The model under review builds one solid part; all positions refer to its coordinate system, in mm. A direction names the side the tool comes from. Give positions to 0.01 mm unless a question says otherwise; leave off trailing zeros. Order: outer loops, then holes, each group sorted by start corner. A loop starts at its lowest first (then second) coordinate and runs counter-clockwise, first axis right, second up. Notation, with made-up numbers: (25.5, 86) - (77.5, 86) arc R28 cw to (77.5, 107) - close; hole circle Ø7 at (69, 67.25). An arc over 180 degrees is marked (long way). Write item = value, one per line. Start each with the question number.
1. Machinability: for faces 5 (the flat face through (20, -31.2, 29)), 6 (the flat face through (14, -76, 0)), 7 (the flat face through (2, -37, 23.3)), 8 (the cylindrical face through (13.619, -62.627, 0.051)), 9 (the flat face through (17, 27, 28)), which of the approach directions +Z, -Z, +X, -X, +Y, -Y give a long, thin tool a straight path to every point of the face, cutting with its end or side? Answer none if there is none.
2. We need section B-B, the plane x = 12. State how many separate pieces and enclosed holes the cut face has, and give its area (3 significant figures).
3. Wall thickness on probe 1 along Z at (x, y) = (8.5, -51); probe 2 along Y at (x, z) = (19.25, 21); probe 3 along Y at (x, z) = (12, 11): over which ranges is each line inside the solid? List them lowest first.
4. We need section A-A, the plane z = 9.8. Give the boundary of the cut face in (x, y).
5. Mouldability with a two-part tool opening along Z and no side actions: class faces 1 (the flat face through (1, -40, -16)), 2 (the flat face through (14, -50, 11.9)), 3 (the flat face through (14, -50, 19.1)), 4 (the flat face through (13, -33, 35)) as pulls with the +Z half, pulls with the -Z half, needs draft (parallel to the pull), parting line crosses it, or undercut.
6. We need section C-C, the plane y = -24. Give the boundary of the cut face in (x, z).
7. For P1, Ø2.5, axis at x = 2, z = 14.5, coming from the -Y side; P2, Ø8.5, axis at x = 17, y = 4.5, coming from the -Z side; P3, Ø8, axis at x = 19, z = -4.5, coming from the +Y side, all flat-tipped, find the tip position at first contact; note any pin that passes through.
from build123d import *

# Parameters (mm, degrees)
SKETCH_1_R          = 35
SKETCH_1_R_2        = 33.5
EXTRUDE_1_DEPTH     = 22
EXTRUDE_START       = -17
EXTRUDE_2_DEPTH     = 17
EXTRUDE_START_2     = -5
EXTRUDE_3_DEPTH     = 5
SKETCH_9_W          = 17
SKETCH_9_H          = 70
EXTRUDE_4_DEPTH     = 5
SKETCH_10_W         = 8
SKETCH_10_H         = 70
EXTRUDE_5_DEPTH     = 2.9
SKETCH_12_W         = 80
SKETCH_12_H         = 80
SKETCH_12_R         = 35
EXTRUDE_7_DEPTH     = 3
SKETCH_3_R          = 1.5
CUT_EXTRUDE_1_DEPTH = 30
CUT_EXTRUDE_3_DEPTH = 15
CUT_EXTRUDE_4_DEPTH = 30
SKETCH_13_R         = 4
CUT_EXTRUDE_5_DEPTH = 3


with BuildPart() as part:
    # 草图1 → 凸台-拉伸1 (new body)
    with BuildSketch(Plane(origin=(0, 0, 0), x_dir=(0, 0, -1), z_dir=(1, 0, 0))):
        Circle(SKETCH_1_R)
        Circle(SKETCH_1_R_2, mode=Mode.SUBTRACT)
    extrude(amount=EXTRUDE_1_DEPTH)

    # 草图2 → 凸台-拉伸2 (add)
    with BuildSketch(Plane(origin=(22, 0, 0), x_dir=(0, 0, -1), z_dir=(1, 0, 0)).offset(EXTRUDE_START)):
        with BuildLine():
            Line((0, -70), (0, -35))
            ThreePointArc((0, -35), (-24.748737342, -24.748737342), (-35, 0))
            Line((-35, 0), (-35, -70))
            Line((-35, -70), (0, -70))
        make_face()
        with BuildLine():
            ThreePointArc((35, 0), (24.748737342, -24.748737342), (0, -35))
            Line((0, -35), (0, -70))
            Line((0, -70), (35, -70))
            Line((35, -70), (35, 0))
        make_face()
    extrude(amount=EXTRUDE_2_DEPTH)

    # 草图4 → 凸台-拉伸3 (add)
    with BuildSketch(Plane(origin=(22, 0, 0), x_dir=(0, 0, -1), z_dir=(1, 0, 0)).offset(EXTRUDE_START_2)):
        with BuildLine():
            Line((35, 35), (0, 35))
            ThreePointArc((0, 35), (24.748737342, 24.748737342), (35, 0))
            Line((35, 0), (35, 35))
        make_face()
        with BuildLine():
            Line((-35, 35), (-35, 0))
            ThreePointArc((-35, 0), (-24.748737342, 24.748737342), (0, 35))
            Line((0, 35), (-35, 35))
        make_face()
    extrude(amount=EXTRUDE_3_DEPTH)

    # 草图9 → 凸台-拉伸4 (add)
    with BuildSketch(Plane.XZ.offset(70)):
        with Locations((13.5, 0)):
            Rectangle(SKETCH_9_W, SKETCH_9_H)
    extrude(amount=EXTRUDE_4_DEPTH)

    # 草图10 → 凸台-拉伸5 (add)
    with BuildSketch(Plane.XZ.offset(75)):
        with Locations((18, 0)):
            Rectangle(SKETCH_10_W, SKETCH_10_H)
    extrude(amount=EXTRUDE_5_DEPTH)

    # 草图12 → 凸台-拉伸7 (add)
    with BuildSketch(Plane.ZY):
        Rectangle(SKETCH_12_W, SKETCH_12_H)
        Circle(SKETCH_12_R, mode=Mode.SUBTRACT)
    extrude(amount=-EXTRUDE_7_DEPTH)

    # 草图3 → 切除-拉伸1 (cut)
    with BuildSketch(Plane(origin=(22, 0, 0), x_dir=(0, 0, -1), z_dir=(1, 0, 0))):
        with BuildLine():
            Line((-30.5, -29), (-30.5, -30.5))
            Line((-30.5, -30.5), (-29, -30.5))
            ThreePointArc((-29, -30.5), (-29.439339828, -29.439339828), (-30.5, -29))
        make_face()
        with BuildLine():
            Line((-29, -30.5), (-30.5, -30.5))
            Line((-30.5, -30.5), (-30.5, -29))
            ThreePointArc((-30.5, -29), (-31.560660172, -31.560660172), (-29, -30.5))
        make_face()
        with BuildLine():
            ThreePointArc((30.5, -29), (29.439339828, -29.439339828), (29, -30.5))
            Line((29, -30.5), (30.5, -30.5))
            Line((30.5, -30.5), (30.5, -29))
        make_face()
        with BuildLine():
            Line((30.5, -30.5), (29, -30.5))
            ThreePointArc((29, -30.5), (30.5, -32), (32, -30.5))
            ThreePointArc((32, -30.5), (31.560660172, -29.439339828), (30.5, -29))
            Line((30.5, -29), (30.5, -30.5))
        make_face()
        with Locations((-30.5, 30.5)):
            Circle(SKETCH_3_R)
        with Locations((30.5, 30.5)):
            Circle(SKETCH_3_R)
    extrude(amount=-CUT_EXTRUDE_1_DEPTH, mode=Mode.SUBTRACT)

    # 草图7 → 切除-拉伸3 (cut)
    with BuildSketch(Plane.ZY.offset(-5)):
        with BuildLine():
            ThreePointArc((-27.25, -30.5), (-28.201902961, -28.201902961), (-30.5, -27.25))
            Line((-30.5, -27.25), (-30.5, -30.5))
            Line((-30.5, -30.5), (-27.25, -30.5))
        make_face()
        with BuildLine():
            Line((-30.5, -30.5), (-30.5, -27.25))
            ThreePointArc((-30.5, -27.25), (-32.798097039, -32.798097039), (-27.25, -30.5))
            Line((-27.25, -30.5), (-30.5, -30.5))
        make_face()
        with BuildLine():
            ThreePointArc((33.75, -30.5), (32.798097039, -28.201902961), (30.5, -27.25))
            Line((30.5, -27.25), (30.5, -30.5))
            Line((30.5, -30.5), (27.25, -30.5))
            ThreePointArc((27.25, -30.5), (30.5, -33.75), (33.75, -30.5))
        make_face()
        with BuildLine():
            Line((30.5, -30.5), (30.5, -27.25))
            ThreePointArc((30.5, -27.25), (28.201902961, -28.201902961), (27.25, -30.5))
            Line((27.25, -30.5), (30.5, -30.5))
        make_face()
    extrude(amount=-CUT_EXTRUDE_3_DEPTH, mode=Mode.SUBTRACT)

    # 草图8 → 切除-拉伸4 (cut)
    with BuildSketch(Plane(origin=(22, 0, 0), x_dir=(0, 0, -1), z_dir=(1, 0, 0))):
        with BuildLine():
            Line((-19.1, -66.389218309), (-19.1, -33.781302014))
            ThreePointArc((-19.1, -33.781302014), (-21.2, -31.681302014), (-23.3, -33.781302014))
            Line((-23.3, -33.781302014), (-23.3, -66.389218309))
            ThreePointArc((-23.3, -66.389218309), (-21.2, -68.489218309), (-19.1, -66.389218309))
        make_face()
        with BuildLine():
            Line((23.3, -66.389218309), (23.3, -33.781302014))
            ThreePointArc((23.3, -33.781302014), (21.2, -31.681302014), (19.1, -33.781302014))
            Line((19.1, -33.781302014), (19.1, -66.389218309))
            ThreePointArc((19.1, -66.389218309), (21.2, -68.489218309), (23.3, -66.389218309))
        make_face()
        with BuildLine():
            Line((-7.7, -62.920659131), (-7.7, -50.420659131))
            Line((-7.7, -50.420659131), (-7.7, -37.920659131))
            ThreePointArc((-7.7, -37.920659131), (-9.8, -35.820659131), (-11.9, -37.920659131))
            Line((-11.9, -37.920659131), (-11.9, -62.920659131))
            ThreePointArc((-11.9, -62.920659131), (-9.8, -65.020659131), (-7.7, -62.920659131))
        make_face()
        with BuildLine():
            Line((2.32685582, -60.300961988), (2.32685582, -40.540356273))
            ThreePointArc((2.32685582, -40.540356273), (0, -38.213500453), (-2.32685582, -40.540356273))
            Line((-2.32685582, -40.540356273), (-2.32685582, -60.300961988))
            ThreePointArc((-2.32685582, -60.300961988), (0, -62.627817808), (2.32685582, -60.300961988))
        make_face()
        with BuildLine():
            Line((11.9, -62.920659131), (11.9, -37.920659131))
            ThreePointArc((11.9, -37.920659131), (9.8, -35.820659131), (7.7, -37.920659131))
            Line((7.7, -37.920659131), (7.7, -50.420659131))
            Line((7.7, -50.420659131), (7.7, -62.920659131))
            ThreePointArc((7.7, -62.920659131), (9.8, -65.020659131), (11.9, -62.920659131))
        make_face()
    extrude(amount=-CUT_EXTRUDE_4_DEPTH, mode=Mode.SUBTRACT)

    # 草图13 → 切除-拉伸5 (cut)
    with BuildSketch(Plane.ZY):
        with Locations((-30.5, -30.5)):
            Circle(SKETCH_13_R)
        with Locations((30.5, -30.5)):
            Circle(SKETCH_13_R)
        with Locations((-30.5, 30.5)):
            Circle(SKETCH_13_R)
        with Locations((30.5, 30.5)):
            Circle(SKETCH_13_R)
    extrude(amount=-CUT_EXTRUDE_5_DEPTH, mode=Mode.SUBTRACT)


solid = part.part
Model answer:
q1.face_5 = -X
q1.face_6 = +Z, -Z, -X, -Y
q1.face_7 = +X, -X, -Y
q1.face_8 = +X, -X
q1.face_9 = +Z, +Y
q2.separate_pieces = 1
q2.enclosed_holes = 8
q2.area = 2,930 mm2
q3.probe_1 = -35 to -23.3, -19.1 to -11.9, -7.7 to -2.33, 2.33 to 7.7, 11.9 to 19.1, 23.3 to 35
q3.probe_2 = -77.9 to -68.48, -31.69 to -26.1, 26.1 to 35
q3.probe_3 = -75 to -64.64, -36.2 to -31.64, 31.64 to 33.23
q4.outline = (0, -35.82) - (3, -35.82) - (3, -33.6) - (5, -33.6) - (5, -35.82) - (22, -35.82) - (22, -32.03) - (0, -32.03) - close; (0, 32.03) - (22, 32.03) - (22, 35) - (17, 35) - (17, 33.6) - (3, 33.6) - (3, 40) - (0, 40) - close; (5, -75) - (14, -75) - (14, -77.9) - (22, -77.9) - (22, -65.02) - (5, -65.02) - close
q5.face_1 = needs draft
q5.face_2 = undercut
q5.face_3 = undercut
q5.face_4 = pulls with the +Z half
q6.outline = (0, -40) - (3, -40) - (3, -25.48) - (5, -25.48) - (5, -35) - (22, -35) - (22, -23.37) - (0, -23.37) - close; (0, 23.37) - (22, 23.37) - (22, 35) - (5, 35) - (5, 25.48) - (3, 25.48) - (3, 40) - (0, 40) - close
q7.P1 = -40
q7.P2 = -35
q7.P3 = 35
